Read the model definition and answer for the solid it produces. Units are mm, in the model's axes. A direction names the side the tool comes from. Round coordinates to 2 decimals unless told otherwise and drop trailing zeros. Order: outer loops, then holes, each group sorted by start corner. A loop starts at its lowest first (then second) coordinate and runs counter-clockwise, first axis right, second up. Notation, with made-up numbers: M 86,21.25 L 105,21.25 A15 ccw 105,36.25 Z; hole C -27,44 d1. An arc over 180 degrees is marked long. Use one line per item in the form item = value. Start each with the question number.
from build123d import *

# Parameters (mm, degrees)
PAD_DEPTH           = 34
PAD001_DEPTH        = 1.6
LINEARPATTERN_COUNT = 2
LINEARPATTERN_PITCH = 32.4
SKETCH_R            = 0.9
POCKET_DEPTH        = 22.001
SKETCH003_W         = 17
SKETCH003_H         = 23.4
POCKET001_DEPTH     = 22.001
FILLET_R            = 1
CHAMFER_SIZE        = 2


with BuildPart() as part:
    # Sketch001 → Pad (new body)
    with BuildSketch(Plane.XZ):
        Polygon((-22, 1.6), (-7.2, 1.6), (-3.2, 5.6), (-3.2, 20), (0, 20), (0, 0), (-22, 0), align=None)
    extrude(amount=PAD_DEPTH)

    # Sketch002 → Pad001 (join)
    with BuildSketch(Plane.XZ):
        Polygon((-6.6, 1.5), (-1.5, 6.6), (-1.5, 1.5), align=None)
    pad001 = extrude(amount=PAD001_DEPTH)

    # LinearPattern: Pad001 ×2
    with Locations(*[(0, -i * LINEARPATTERN_PITCH, 0) for i in range(1, LINEARPATTERN_COUNT)]):
        add(pad001)

    # Sketch (on DatumPlane) → Pocket (cut, through all)
    with BuildSketch(Plane(origin=(0, 0, 0), x_dir=(0, 0, 1), z_dir=(1, 0, 0))):
        with Locations((16.6, 30.8)):
            Circle(SKETCH_R)
        with Locations((16.6, 3.6)):
            Circle(SKETCH_R)
    extrude(amount=-POCKET_DEPTH, mode=Mode.SUBTRACT)

    # Sketch003 (on DatumPlane) → Pocket001 (cut, through all)
    with BuildSketch(Plane(origin=(0, 0, 0), x_dir=(0, 0, 1), z_dir=(1, 0, 0))):
        with Locations((13.5, 17.2)):
            Rectangle(SKETCH003_W, SKETCH003_H)
    extrude(amount=-POCKET001_DEPTH, mode=Mode.SUBTRACT)

    # Fillet
    fillet_edges = [part.edges().sort_by_distance(p)[0] for p in [
        (-1.6, -34, 20),
        (-1.6, -28.9, 20),
        (-1.6, -5.5, 20),
        (-1.6, 0, 20),
    ]]
    fillet(fillet_edges, radius=FILLET_R)

    # Chamfer
    chamfer_edges = [part.edges().sort_by_distance(p)[0] for p in [
        (-1.9, -28.9, 5),
        (-1.9, -5.5, 5),
    ]]
    chamfer(chamfer_edges, length=CHAMFER_SIZE)


solid = part.part
Item 1: For a pull along Y with two mould halves and no side action, classify faces 3 (the flat face through (-1.9, -27.9, 6)), 4 (the cylindrical face through (-1.622, -29.185, 19.699)), 5 (the flat face through (-5.2, -16.8, 3.6)), 6 (the flat face through (-3, -34, 7)) as pulls with the +Y half, pulls with the -Y half, needs draft (parallel to the pull), parting line crosses it, or undercut.
Item 2: Given P1, Ø5.5, axis at y = -3, z = 16, coming from the -X side; P2, Ø4, axis at x = -5, y = -13.5, coming from the +Z side; P3, Ø10, axis at x = -17.5, y = -23.5, coming from the +Z side, each flat-ended and moving along its own axis, determine where each tip first touches the part or whether it passes through.
Item 3: Section A-A (y = -3.6) is taken. Write down the section's boundary in (x, z), and give its area (3 significant figures).
Item 4: Section C-C (z = 16.6) is taken. Write down the section's boundary in (x, y).
Item 5: Find the intervals of material crossed by L1, parallel to Y at x = -1.7, z = 16.6; L2, parallel to Z at x = -2.5, y = -3.6; L3, parallel to Z at x = -8.5, y = -19, in increasing order. Write a range as [from, to].
Item 6: A tool of negligible diameter and unlimited length cuts with its end or side. For faces 1 (the flat face through (-2, -5.5, 13)), 2 (the cylindrical face through (-1.578, -33.715, 19.699)), from which of +Z, -Z, +X, -X, +Y, -Y can it reach the whole face along a straight path? Write none if from no direction.
Item 7: Section D-D (y = -10.5) is taken. Write down the section's boundary in (x, z), and give its area (3 significant figures).
Item 8: Section B-B (z = 6) is taken. Write down the section's boundary in (x, y).
The answers:
q1.face_3 = undercut
q1.face_4 = undercut
q1.face_5 = needs draft
q1.face_6 = pulls with the -Y half
q2.P1 = -3.2
q2.P2 = 5
q2.P3 = 1.6
q3.outline = M -22,0 L 0,0 L 0,15.7 L -3.2,15.7 L -3.2,5.6 L -7.2,1.6 L -22,1.6 Z; M -3.2,17.5 L 0,17.5 L 0,20 L -3.2,20 Z
q3.area = 96.3 mm²
q4.outline = M -3.2,-34 L 0,-34 L 0,-31.7 L -3.2,-31.7 Z; M -3.2,-29.9 L 0,-29.9 L 0,-28.9 L -3.2,-28.9 Z; M -3.2,-5.5 L 0,-5.5 L 0,-4.5 L -3.2,-4.5 Z; M -3.2,-2.7 L 0,-2.7 L 0,0 L -3.2,0 Z
q5.L1 = [-34, -31.7], [-29.9, -28.9], [-5.5, -4.5], [-2.7, 0]
q5.L2 = [0, 15.7], [17.5, 20]
q5.L3 = [0, 1.6]
q6.face_1 = +Z, +X, -X
q6.face_2 = +Z, +X, -X, -Y
q7.outline = M -22,0 L 0,0 L 0,5 L -3.8,5 L -7.2,1.6 L -22,1.6 Z
q7.area = 53.9 mm²
q8.outline = M -3.2,-34 L 0,-34 L 0,-27.9 L -3.2,-27.9 Z; M -3.2,-6.5 L 0,-6.5 L 0,0 L -3.2,0 Z
